Check sheet for the modelled part. Datum: model origin and axes. Units: mm. Round coordinates to 2 decimals unless told otherwise and drop trailing zeros. Order: outer loops, then holes, each group sorted by start corner. A loop starts at its lowest first (then second) coordinate and runs counter-clockwise, first axis right, second up. Notation, with made-up numbers: (10, 66.25) -> (69, 66.25) arc R30 ccw to (69, 103.25) -> close; hole circle Ø5 at (-19, 78). An arc over 180 degrees is marked (long way). Answer in a Markdown table with one row per item. Add a question column.
1. Depth check by flat-ended pin: P1, Ø4, axis at y = -10.5, z = -168.5, coming from the -X side; P2, Ø6, axis at x = 276.5, y = -7, coming from the -Z side; P3, Ø6, axis at x = 115.5, y = -11, coming from the -Z side. Enter the tip coordinate at first touch or a pass-through.
2. Sectioned sample at C-C, the plane x = 45. Record the boundary of the cut face in (y, z), then the cut area to 3 significant figures.
3. Sectioned sample at A-A, the plane z = -202. Record the boundary of the cut face in (x, y).
4. Material ranges on L1, parallel to X at y = -11, z = -60.5; L2, parallel to X at y = -12.75, z = -105.5; L3, parallel to X at y = -2.25, z = -664, recorded low to high. Write a range as from..to.
5. Sectioned sample at B-B, the plane x = 199. Record the boundary of the cut face in (y, z), then the cut area to 3 significant figures.
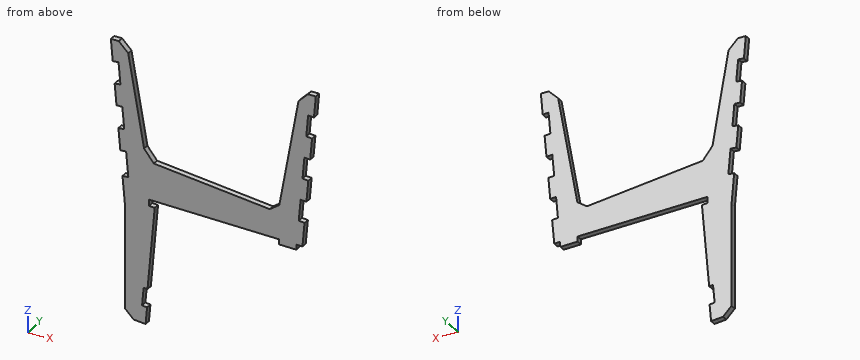
```python
from build123d import *
from OCP.BRepFilletAPI import BRepFilletAPI_MakeChamfer

# Parameters (mm, degrees)
BOSS_EXTRUDE1_DEPTH = 15
CUT_EXTRUDE2_DEPTH  = 816.748946497
BOSS_EXTRUDE2_DEPTH = 15
BOSS_EXTRUDE3_DEPTH = 15
CHAMFER1_SIZE       = 20
CHAMFER1_SIZE2      = 22.009925117
CHAMFER2_SIZE       = 20
CHAMFER2_SIZE2      = 21.383906801
CHAMFER2_SIZE2_2    = 29.545676359
CHAMFER3_SIZE       = 20
CHAMFER3_SIZE2      = 24.656061036
CUT_EXTRUDE3_DEPTH  = 817.728441489


with BuildPart() as part:
    # Sketch3 → Boss-Extrude1 (new body)
    with BuildSketch(Plane(origin=(0, 0, 0), x_dir=(1, 0, 0), z_dir=(0, 1, 0))):
        Polygon((410, 0), (375.499079338, 394.347327661), (-3.698775856, 385.063270846), (-23.780817684, 615.47886016), (-33.743052085, 614.610594222), (-41.626962847, 705.068325562), (-61.474466641, 703.331893981), (-81.398360603, 701.588779126), (-81.491356741, 420.124681698), (-118.247503657, 0), (-77.901012172, 0), (-27.385966046, 286.485062711), (312.415130717, 324.614971391), (369.653508515, 0), align=None)
    extrude(amount=-BOSS_EXTRUDE1_DEPTH)

    # Sketch4 → Cut-Extrude2 (cut, through all)
    with BuildSketch(Plane(origin=(0, 0, 0), x_dir=(1, 0, 0), z_dir=(0, 1, 0))):
        Polygon((-20.036108533, 401.037382744), (-19.638496356, 384.673012123), (-3.698775856, 385.063270846), (-5.122834429, 401.402510558), align=None)
    extrude(amount=-CUT_EXTRUDE2_DEPTH, mode=Mode.SUBTRACT)

    # Sketch5 → Boss-Extrude2 (add)
    with BuildSketch(Plane(origin=(0, 0, 0), x_dir=(1, 0, 0), z_dir=(0, 1, 0))):
        Polygon((-41.626962847, 705.068325562), (-28.676431065, 706.20135028), (-24.852581449, 662.327596289), (-37.80348617, 661.198850569), align=None)
    extrude(amount=-BOSS_EXTRUDE2_DEPTH)

    # Sketch6 → Boss-Extrude3 (add)
    with BuildSketch(Plane(origin=(0, 0, 0), x_dir=(1, 0, 0), z_dir=(0, 1, 0))):
        Polygon((315.438962688, 392.87685116), (360.503573098, 393.980186523), (359.842168491, 407.025169305), (315.461186161, 405.938571489), align=None)
    extrude(amount=-BOSS_EXTRUDE3_DEPTH)

    # Chamfer1
    chamfer1_edges = [part.edges().sort_by_distance(p)[0] for p in [
        (-81.398360603, -7.5, -701.588779126),
    ]]
    chamfer1_side = [part.faces().sort_by_distance(p)[0] for p in [
        (-81.444858672, -7.5, -560.856730412),
    ]]
    chamfer(chamfer1_edges, length=CHAMFER1_SIZE, length2=CHAMFER1_SIZE2, reference=chamfer1_side[0])

    # Chamfer2: one chamfer whose edges measure the first distance from different faces: ONE call of the kernel's chamfer builder (chamfer() names one face for all edges)
    chamfer2_edges_1 = [part.edges().sort_by_distance(p)[0] for p in [
        (312.415130717, -7.5, -324.614971391),
    ]]
    chamfer2_side_1 = [part.faces().sort_by_distance(p)[0] for p in [
        (341.034319616, -7.5, -162.307485695),
    ]]
    chamfer2_edges_2 = [part.edges().sort_by_distance(p)[0] for p in [
        (-27.385966046, -7.5, -286.485062711),
    ]]
    chamfer2_side_2 = [part.faces().sort_by_distance(p)[0] for p in [
        (142.514582336, -7.5, -305.550017051),
    ]]
    chamfer2 = BRepFilletAPI_MakeChamfer(part.part.solid().wrapped)
    for e in chamfer2_edges_1:
        chamfer2.Add(CHAMFER2_SIZE, CHAMFER2_SIZE2, e.wrapped, chamfer2_side_1[0].wrapped)  # the first distance lies on this face
    for e in chamfer2_edges_2:
        chamfer2.Add(CHAMFER2_SIZE, CHAMFER2_SIZE2_2, e.wrapped, chamfer2_side_2[0].wrapped)  # the first distance lies on this face
    add(Compound.cast(chamfer2.Shape()), mode=Mode.REPLACE)

    # Chamfer3: one chamfer whose edges measure the first distance from different faces: ONE call of the kernel's chamfer builder (chamfer() names one face for all edges)
    chamfer3_edges_1 = [part.edges().sort_by_distance(p)[0] for p in [
        (369.653508515, -7.5, 0),
    ]]
    chamfer3_side_1 = [part.faces().sort_by_distance(p)[0] for p in [
        (389.826754258, -7.5, 0),
    ]]
    chamfer3_edges_2 = [part.edges().sort_by_distance(p)[0] for p in [
        (-77.901012172, -7.5, 0),
    ]]
    chamfer3_side_2 = [part.faces().sort_by_distance(p)[0] for p in [
        (-98.074257914, -7.5, 0),
    ]]
    chamfer3 = BRepFilletAPI_MakeChamfer(part.part.solid().wrapped)
    for e in chamfer3_edges_1:
        chamfer3.Add(CHAMFER3_SIZE, CHAMFER3_SIZE2, e.wrapped, chamfer3_side_1[0].wrapped)  # the first distance lies on this face
    for e in chamfer3_edges_2:
        chamfer3.Add(CHAMFER3_SIZE, CHAMFER3_SIZE2, e.wrapped, chamfer3_side_2[0].wrapped)  # the first distance lies on this face
    add(Compound.cast(chamfer3.Shape()), mode=Mode.REPLACE)

    # Sketch9 → Cut-Extrude3 (cut, through all)
    with BuildSketch(Plane(origin=(0, 0, 0), x_dir=(1, 0, 0), z_dir=(0, 1, 0))):
        Polygon((-73.280468193, 341.864865291), (-78.892311228, 277.721205877), (-93.835666105, 279.028580024), (-88.223823069, 343.172239438), align=None)
        Polygon((-98.717946571, 223.223858938), (-83.774591695, 221.916484791), (-88.656865511, 166.111839714), (-103.714600804, 166.111839714), align=None)
        Polygon((-93.539152627, 110.307042618), (-108.482507504, 111.614416765), (-113.36478797, 55.809695678), (-98.421433094, 54.502321532), align=None)
        Polygon((380.927264722, 332.302884814), (365.983909846, 330.995510667), (370.829365725, 275.611696532), (385.772720602, 276.919070678), align=None)
        Polygon((390.618176481, 221.535256543), (375.674821605, 220.227882396), (380.520277485, 164.84406826), (395.463632361, 166.151442407), align=None)
        Polygon((385.365733364, 109.460254125), (390.211189244, 54.076439989), (405.15454412, 55.383814136), (400.309088241, 110.767628271), align=None)
    extrude(amount=-CUT_EXTRUDE3_DEPTH, mode=Mode.SUBTRACT)


solid = part.part
```
Answer key:
| question | item | result |
|---|---|---|
| 1 | P1 | stops at x = -88.62 |
| 1 | P2 | stops at z = -392 |
| 1 | P3 | stops at z = -388.06 |
| 2 | outline | (-15, -386.26) -> (0, -386.26) -> (0, -294.61) -> (-15, -294.61) -> close |
| 2 | area | 1,370 mm² |
| 3 | outline | (-85.52, -15) -> (-42.28, -15) -> (-42.28, 0) -> (-85.52, 0) -> close; (334.04, -15) -> (377.27, -15) -> (377.27, 0) -> (334.04, 0) -> close |
| 4 | L1 | x = -97.9..-67.23, 358.99..389.65 |
| 4 | L2 | x = -93.96..-59.3, 351.05..385.71 |
| 4 | L3 | x = -81.41..-25 |
| 5 | outline | (-15, -390.03) -> (0, -390.03) -> (0, -311.89) -> (-15, -311.89) -> close |
| 5 | area | 1,170 mm² |
